Work out the finished part from the listing and answer in its coordinate system (mm). A direction names the side the tool comes from. Give positions to 0.01 mm unless a question says otherwise; leave off trailing zeros. Write each loop counter-clockwise with the first axis right and the second up, starting at its lowest first coordinate (ties: lowest second). Pieces come first, ordered by that corner, then holes. Notation, with made-up numbers: (-16.5, 33) -> (13.5, 33) arc R5 ccw to (13.5, 40) -> close; hole circle Ø1 at (43.5, -16.5). An arc over 180 degrees is marked (long way). Use a Markdown table: item, result. Add a question column.
Q1. Section B-B, the plane z = 3.5 is taken. Give the vertices of the cut face in (x, y), plus the area to 3 significant figures.
Q2. Consider line 1 (X direction, y = 3.45, z = -38); line 2 (Z direction, x = -65, y = 3.4); line 3 (Z direction, x = -60.5, y = 4.85). Determine where each line is inside the solid, lowest interval first.
Q3. This flat-tipped pin is pushed along its axis until it touches: pin 1 Ø1.5 at (y, z) = (2, -58) entering from -X. Where does it stop, or does it pass through?
Q4. For faces 5 (the face through (-1, 2, 70)), 6 (the face through (-52.5, 3, 0)), determine the directions among +Z, -Z, +X, -X, +Y, -Y from which every point of the face is accessible in a straight line to the end or side of a thin tool.
Q5. Section A-A, the plane x = -3.5 is taken. Give the vertices of the cut face in (y, z), plus the area to 3 significant figures.
Q6. Section C-C, the plane y = 3.5 is taken. State how many separate pieces and enclosed holes the cut face has, plus the area to 3 significant figures.
Q7. For a pull along X with two mould halves and no side action, classify faces 1 (the face through (0, 3, -58.336)), 2 (the face through (-77.5, 2, 1)), 3 (the face through (73.793, 2.535, 66.091)), 4 (the face through (-58, 3, -49)) as pulls with the +X half, pulls with the -X half, needs draft (parallel to the pull), parting line crosses it, or undercut.
from build123d import *

# Parameters (mm, degrees)
SKETCH1_W           = 155
SKETCH1_H           = 140
BOSS_EXTRUDE1_DEPTH = 5
CUT_EXTRUDE1_DEPTH  = 5
SKETCH3_R           = 1.4
CUT_EXTRUDE2_DEPTH  = 5
SKETCH5_W           = 60
SKETCH5_H           = 10
CUT_EXTRUDE3_DEPTH  = 5
SKETCH6_R           = 1.4
CUT_EXTRUDE4_DEPTH  = 10
SKETCH7_W           = 15
SKETCH7_H           = 25
CUT_EXTRUDE5_DEPTH  = 10
SKETCH8_W           = 19.2
SKETCH8_H           = 13
CUT_EXTRUDE6_DEPTH  = 10
FILLET2_R           = 2
FILLET3_R           = 2


with BuildPart() as part:
    # Sketch1 → Boss-Extrude1 (new body)
    with BuildSketch(Plane(origin=(0, 0, 0), x_dir=(1, 0, 0), z_dir=(0, 1, 0))):
        Rectangle(SKETCH1_W, SKETCH1_H)
    extrude(amount=BOSS_EXTRUDE1_DEPTH)

    # Sketch2 → Cut-Extrude1 (cut)
    with BuildSketch(Plane(origin=(0, 5, 0), x_dir=(1, 0, 0), z_dir=(0, 1, 0))):
        with BuildLine():
            Line((-77.5, 70), (-77.5, 57))
            ThreePointArc((-77.5, 57), (-73.692388155, 66.192388155), (-64.5, 70))
            Line((-64.5, 70), (-77.5, 70))
        make_face()
        with BuildLine():
            Line((77.5, 70), (64.5, 70))
            ThreePointArc((64.5, 70), (73.692388155, 66.192388155), (77.5, 57))
            Line((77.5, 57), (77.5, 70))
        make_face()
        with BuildLine():
            Line((77.5, -70), (77.5, -57))
            ThreePointArc((77.5, -57), (73.692388155, -66.192388155), (64.5, -70))
            Line((64.5, -70), (77.5, -70))
        make_face()
        with BuildLine():
            Line((-77.5, -70), (-64.5, -70))
            ThreePointArc((-64.5, -70), (-73.692388155, -66.192388155), (-77.5, -57))
            Line((-77.5, -57), (-77.5, -70))
        make_face()
    extrude(amount=-CUT_EXTRUDE1_DEPTH, mode=Mode.SUBTRACT)

    # Sketch3 → Cut-Extrude2 (cut)
    with BuildSketch(Plane(origin=(0, 5, 0), x_dir=(1, 0, 0), z_dir=(0, 1, 0))):
        with Locations(Location((-65, 38, 0), (0, 0, 270))):
            Circle(SKETCH3_R)
        with Locations(Location((65, 38, 0), (0, 0, 90))):
            Circle(SKETCH3_R)
        with Locations(Location((65, -50, 0), (0, 0, 270))):
            Circle(SKETCH3_R)
        with Locations(Location((-65, -50, 0), (0, 0, 90))):
            Circle(SKETCH3_R)
    extrude(amount=-CUT_EXTRUDE2_DEPTH, mode=Mode.SUBTRACT)

    # Sketch5 → Cut-Extrude3 (cut)
    with BuildSketch(Plane(origin=(0, 5, 0), x_dir=(1, 0, 0), z_dir=(0, 1, 0))):
        with Locations((0, 53.335629909)):
            Rectangle(SKETCH5_W, SKETCH5_H)
    extrude(amount=-CUT_EXTRUDE3_DEPTH, mode=Mode.SUBTRACT)

    # Sketch6 → Cut-Extrude4 (cut)
    with BuildSketch(Plane(origin=(0, 5, 0), x_dir=(1, 0, 0), z_dir=(0, 1, 0))):
        with Locations(Location((-17, -40, 0), (0, 0, 270))):
            Circle(SKETCH6_R)
        with Locations(Location((17, -40, 0), (0, 0, 270))):
            Circle(SKETCH6_R)
        with Locations(Location((17, -60, 0), (0, 0, 270))):
            Circle(SKETCH6_R)
        with Locations(Location((-17, -60, 0), (0, 0, 270))):
            Circle(SKETCH6_R)
    extrude(amount=-CUT_EXTRUDE4_DEPTH, mode=Mode.SUBTRACT)

    # Sketch7 → Cut-Extrude5 (cut)
    with BuildSketch(Plane(origin=(0, 5, 0), x_dir=(1, 0, 0), z_dir=(0, 1, 0))):
        with Locations((-60, 0)):
            Rectangle(SKETCH7_W, SKETCH7_H)
    extrude(amount=-CUT_EXTRUDE5_DEPTH, mode=Mode.SUBTRACT)

    # Sketch8 → Cut-Extrude6 (cut)
    with BuildSketch(Plane(origin=(0, 5, 0), x_dir=(1, 0, 0), z_dir=(0, 1, 0))):
        with Locations((-57.9, 55.5)):
            Rectangle(SKETCH8_W, SKETCH8_H)
    extrude(amount=-CUT_EXTRUDE6_DEPTH, mode=Mode.SUBTRACT)

    # Fillet2
    fillet2_edges = [part.edges().sort_by_distance(p)[0] for p in [
        (-52.5, 2.5, -12.5),
        (-52.5, 2.5, 12.5),
        (-67.5, 2.5, 12.5),
        (-67.5, 2.5, -12.5),
    ]]
    fillet(fillet2_edges, radius=FILLET2_R)

    # Fillet3
    fillet3_edges = [part.edges().sort_by_distance(p)[0] for p in [
        (30, 2.5, -58.335629909),
        (30, 2.5, -48.335629909),
        (-30, 2.5, -48.335629909),
        (-30, 2.5, -58.335629909),
    ]]
    fillet(fillet3_edges, radius=FILLET3_R)


solid = part.part
Result set:
| question | item | result |
|---|---|---|
| 1 | outline | (-77.5, 0) -> (-67.5, 0) -> (-67.5, 5) -> (-77.5, 5) -> close; (-52.5, 0) -> (77.5, 0) -> (77.5, 5) -> (-52.5, 5) -> close |
| 1 | area | 700 mm2 |
| 2 | line 1 | x = -77.5 to -66.4, -63.6 to 63.6, 66.4 to 77.5 |
| 2 | line 2 | z = -69.99 to -62, -49 to -39.4, -36.6 to -12.5, 12.5 to 48.6, 51.4 to 69.99 |
| 2 | line 3 | z = -70 to -62, -49 to -12.5, 12.5 to 70 |
| 3 | pin 1 | stops at x = -77.5 |
| 4 | face 5 | +Z, +X, -X, +Y, -Y |
| 4 | face 6 | +Y, -Y |
| 5 | outline | (0, -70) -> (5, -70) -> (5, -58.34) -> (0, -58.34) -> close; (0, -48.34) -> (5, -48.34) -> (5, 70) -> (0, 70) -> close |
| 5 | area | 650 mm2 |
| 6 | separate pieces | 1 |
| 6 | enclosed holes | 11 |
| 6 | area | 20,300 mm2 |
| 7 | face 1 | undercut |
| 7 | face 2 | pulls with the -X half |
| 7 | face 3 | pulls with the +X half |
| 7 | face 4 | undercut |
